Verification items for the finished model (mm, model axes). Face numbers are marked on the shaded views. A direction names the side the tool comes from. Round coordinates to 2 decimals unless told otherwise and drop trailing zeros. Write each loop counter-clockwise with the first axis right and the second up, starting at its lowest first coordinate (ties: lowest second). Pieces come first, ordered by that corner, then holes. Notation, with made-up numbers: M 21.5,0 L 35.5,0 A14 ccw 35.5,20 Z; hole C 14.5,-15 d10. An arc over 180 degrees is marked long. One line per item, written item: value. Start each with the question number.
Item 1: Gauge pin test, flat ends, axial feed: pin 1 (1.9 mm diameter, centred on x = -4, y = 21, fed in from +Z) (3 decimals); pin 2 (6.5 mm diameter, centred on y = -2, z = 1.5, fed in from -X); pin 3 (4.5 mm diameter, centred on x = -7.5, z = -0.5, fed in from +Y); pin 4 (5 mm diameter, centred on y = -2.5, z = -10, fed in from -X). Record the tip position at first contact, or that the pin passes through.
Item 2: Section check C-C, the plane x = 3. Record the cut outline in (y, z), then the cut area to 3 significant figures.
Item 3: Tool access check on the marked faces 1, 2, 3, 4 and 5. Record the directions out of +Z, -Z, +X, -X, +Y, -Y that give a thin tool (end or side, any length) a straight path to the whole face; none if there is none.
Item 4: Thickness scan on probe 1 along Y at (x, z) = (18.5, 0); probe 2 along Y at (x, z) = (1, 0); probe 3 along X at (y, z) = (-3, -9.75). Record the ranges inside material, lowest first. Write a range as from..to.
Item 5: Section check A-A, the plane x = 14. Record the cut outline in (y, z).
Item 6: Draft check along Z on the marked faces 6, 7, 8 and 9. Enter one of: +Z half, -Z half, draft (parallel to the pull), parting line (faces both ways), or undercut.
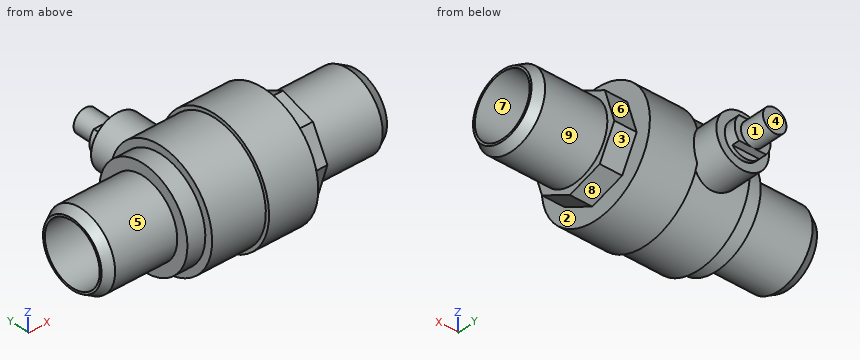
from build123d import *

# Parameters (mm, degrees)
SKETCH1_R               = 8.46455
BOSS_EXTRUDE1_DEPTH     = 31.89
BOSS_EXTRUDE3_DEPTH     = 5
SKETCH6_R               = 13.5
BOSS_EXTRUDE4_DEPTH     = 11
SKETCH7_R               = 12.7
BOSS_EXTRUDE5_DEPTH     = 12
SKETCH8_R               = 11
BOSS_EXTRUDE6_DEPTH     = 4
SKETCH9_R               = 5.875
BOSS_EXTRUDE7_DEPTH     = 19.1
SKETCH10_R              = 4
BOSS_EXTRUDE8_DEPTH     = 2.5
SKETCH11_OUTSIDE_W      = 81.31
SKETCH11_OUTSIDE_H      = 44.53
SKETCH11_OUTSIDE_W_2    = 14.822508056
SKETCH11_OUTSIDE_H_2    = 5.25
CUT_EXTRUDE4_DEPTH      = 1.7
SKETCH12_R              = 2.625
BOSS_EXTRUDE9_DEPTH     = 5.5
SKETCH2_R               = 6.84
CUT_EXTRUDE3_DEPTH      = 32.89
CUT_EXTRUDE3_DEPTH_BACK = 32.89
CHAMFER1_SIZE           = 2
CHAMFER1_SIZE2          = 1.154700538
CHAMFER1_PART_2_SIZE    = 2
CHAMFER1_PART_2_SIZE2   = 1.154700538


with BuildPart() as part:
    # Sketch1 → Boss-Extrude1 (new body, symmetric)
    with BuildSketch(Plane(origin=(0, 0, 0), x_dir=(0, 0, -1), z_dir=(1, 0, 0))):
        Circle(SKETCH1_R)
    extrude(amount=BOSS_EXTRUDE1_DEPTH, both=True)

    # Sketch5 → Boss-Extrude3 (add)
    with BuildSketch(Plane(origin=(15.99, 0, 0), x_dir=(0, 0, -1), z_dir=(1, 0, 0))):
        Polygon((7.845102358, 6.582822495), (0.892566651, 10.202083501), (-6.582822495, 7.845102358), (-10.202083501, 0.892566651), (-7.845102358, -6.582822495), (-0.892566651, -10.202083501), (6.582822495, -7.845102358), (10.202083501, -0.892566651), align=None)
    extrude(amount=-BOSS_EXTRUDE3_DEPTH)

    # Sketch6 → Boss-Extrude4 (add)
    with BuildSketch(Plane.ZY.offset(-10.99)):
        Circle(SKETCH6_R)
    extrude(amount=BOSS_EXTRUDE4_DEPTH)

    # Sketch7 → Boss-Extrude5 (add)
    with BuildSketch(Plane.ZY.offset(0.01)):
        Circle(SKETCH7_R)
    extrude(amount=BOSS_EXTRUDE5_DEPTH)

    # Sketch8 → Boss-Extrude6 (add)
    with BuildSketch(Plane.ZY.offset(12.01)):
        Circle(SKETCH8_R)
    extrude(amount=BOSS_EXTRUDE6_DEPTH)

    # Sketch9 → Boss-Extrude7 (add)
    with BuildSketch(Plane(origin=(0, 0, 0), x_dir=(1, 0, 0), z_dir=(0, 1, 0))):
        with Locations((-4.715, 0)):
            Circle(SKETCH9_R)
    extrude(amount=BOSS_EXTRUDE7_DEPTH)

    # Sketch10 → Boss-Extrude8 (add)
    with BuildSketch(Plane(origin=(0, 19.1, 0), x_dir=(1, 0, 0), z_dir=(0, 1, 0))):
        with Locations((-4.715, 0)):
            Circle(SKETCH10_R)
    extrude(amount=BOSS_EXTRUDE8_DEPTH)

    # Sketch11 outside → Cut-Extrude4 (cut)
    with BuildSketch(Plane(origin=(0, 21.6, 0), x_dir=(1, 0, 0), z_dir=(0, 1, 0))):
        Rectangle(SKETCH11_OUTSIDE_W, SKETCH11_OUTSIDE_H)
        with Locations((-4.715, 0)):
            Rectangle(SKETCH11_OUTSIDE_W_2, SKETCH11_OUTSIDE_H_2, mode=Mode.SUBTRACT)
    extrude(amount=-CUT_EXTRUDE4_DEPTH, mode=Mode.SUBTRACT)

    # Sketch12 → Boss-Extrude9 (add)
    with BuildSketch(Plane(origin=(0, 21.6, 0), x_dir=(1, 0, 0), z_dir=(0, 1, 0))):
        with Locations((-4.715, 0)):
            Circle(SKETCH12_R)
    extrude(amount=BOSS_EXTRUDE9_DEPTH)

    # Sketch2 → Cut-Extrude3 (cut, two sides)
    with BuildSketch(Plane(origin=(0, 0, 0), x_dir=(0, 0, -1), z_dir=(1, 0, 0))) as cut_extrude3_sk:
        Circle(SKETCH2_R)
    extrude(amount=CUT_EXTRUDE3_DEPTH, mode=Mode.SUBTRACT)
    extrude(cut_extrude3_sk.sketch, amount=-CUT_EXTRUDE3_DEPTH_BACK, mode=Mode.SUBTRACT)

    # Chamfer1
    chamfer1_edges = [part.edges().sort_by_distance(p)[0] for p in [
        (-31.89, 0, 8.46455),
    ]]
    chamfer1_side = [part.faces().sort_by_distance(p)[0] for p in [
        (-23.95, 0, 8.46455),
    ]]
    chamfer(chamfer1_edges, length=CHAMFER1_SIZE, length2=CHAMFER1_SIZE2, reference=chamfer1_side[0])

    # Chamfer1 part 2
    chamfer1_part_2_edges = [part.edges().sort_by_distance(p)[0] for p in [
        (31.89, 0, 8.46455),
    ]]
    chamfer1_part_2_side = [part.faces().sort_by_distance(p)[0] for p in [
        (23.94, 0, 8.46455),
    ]]
    chamfer(chamfer1_part_2_edges, length=CHAMFER1_PART_2_SIZE, length2=CHAMFER1_PART_2_SIZE2, reference=chamfer1_part_2_side[0])


solid = part.part
Response values:
1. pin 1: stops at z = 2.625
1. pin 2: passes through
1. pin 3: stops at y = 27.1
1. pin 4: stops at x = -31.03
2. outline: C 0,0 d27; hole C 0,0 d13.68
2. area: 426 mm2
3. face 1: +Y
3. face 2: +X
3. face 3: -Z, +X, +Y
3. face 4: +Z, -Z, +X, -X, +Y
3. face 5: -X
4. probe 1: y = -8.46..-6.84, 6.84..8.46
4. probe 2: y = -13.5..-6.84, 6.84..19.1
4. probe 3: x = -16.01..10.99
5. outline: M -10.2,0.89 L -7.85,-6.58 L -0.89,-10.2 L 6.58,-7.85 L 10.2,-0.89 L 7.85,6.58 L 0.89,10.2 L -6.58,7.85 Z; hole C 0,0 d13.68
6. face 6: +Z half
6. face 7: undercut
6. face 8: -Z half
6. face 9: parting line
